```python
from build123d import *

# Parameters (mm, degrees)
PAD_DEPTH   = 5.5
FILLET_R    = 0.3
FILLET001_R = 0.3


with BuildPart() as part:
    # Sketch → Pad (new body)
    with BuildSketch(Plane.XY):
        Polygon((-10, 1.5), (10, 1.5), (10, -3.2), (8.5, -3.2), (7.5, -2), (8.5, -2), (8.5, 0), (-8.5, 0), (-8.5, -2), (-7.5, -2), (-8.5, -3.2), (-10, -3.2), align=None)
    extrude(amount=PAD_DEPTH)

    # Fillet
    fillet_edges = [part.edges().sort_by_distance(p)[0] for p in [
        (-7.5, -2, 2.75),
    ]]
    fillet(fillet_edges, radius=FILLET_R)

    # Fillet001
    fillet001_edges = [part.edges().sort_by_distance(p)[0] for p in [
        (7.5, -2, 2.75),
    ]]
    fillet(fillet001_edges, radius=FILLET001_R)


solid = part.part
```
Design review of the part built by this model. Coordinates are the model's own, in mm. Round coordinates to 2 decimals unless told otherwise and drop trailing zeros. Write each loop counter-clockwise with the first axis right and the second up, starting at its lowest first coordinate (ties: lowest second). Pieces come first, ordered by that corner, then holes.
Item 1: The part is to be moulded in two halves that separate along Y. For faces 1 (the flat face through (0, 1.5, 3)), 2 (the flat face through (8.5, -1, 3)), 3 (the flat face through (-8.5, -1, 3)), 4 (the flat face through (-9, -3.2, 3)), say which applies: +Y half, -Y half, draft (parallel to the pull), parting line (faces both ways), or undercut.
Item 2: For probe 1 along X at (y, z) = (-0.05, 1.9); probe 2 along Y at (x, z) = (1.25, 2.3); probe 3 along Y at (x, z) = (8, 4.8), list the stretches that pass through material, from the lowest coordinate up.
Item 3: We need section A-A on z = 2.85. Write out the cut boundary in (x, y).
Item 4: We need section B-B on x = 3.5. Write out the cut boundary in (y, z).
Item 5: Clearance check with a flat-ended pin moving along its axis: pin 1 Ø1.5 at (x, y) = (3.5, -1.5) entering from -Z. State where the tip first meets the part, or that it passes through.
Returned:
1. face 1: +Y half
1. face 2: undercut
1. face 3: undercut
1. face 4: -Y half
2. probe 1: x = -10 to -8.5, 8.5 to 10
2. probe 2: y = 0 to 1.5
2. probe 3: y = -2.6 to -2.03, 0 to 1.5
3. outline: (-10, -3.2) - (-8.5, -3.2) - (-7.91, -2.49) arc R0.3 ccw to (-8.14, -2) - (-8.5, -2) - (-8.5, 0) - (8.5, 0) - (8.5, -2) - (8.14, -2) arc R0.3 ccw to (7.91, -2.49) - (8.5, -3.2) - (10, -3.2) - (10, 1.5) - (-10, 1.5) - close
4. outline: (0, 0) - (1.5, 0) - (1.5, 5.5) - (0, 5.5) - close
5. pin 1: passes through
